Autodesk Inventor part; units mm, degrees
ref_plane "YZ Plane" through (0, 0, 0) normal (1, 0, 0) x (0, 1, 0)
ref_plane "XZ Plane" through (0, 0, 0) normal (0, 1, 0) x (-1, 0, 0)
ref_plane "XY Plane" through (0, 0, 0) normal (0, 0, 1) x (1, 0, 0)
sketch "Sketch1" plane through (0, 0, 0) normal (0, 0, 1) x (1, 0, 0)
  line L0 (-750, 62.1281) -> (750, 62.1281)
  line L1 (750, 62.1281) -> (750, 0)
  line L2 (750, 0) -> (-750, 0)
  line L3 (-750, 0) -> (-750, 62.1281)
  point P0 (0, 0)
  point P1 (0, 0)
  dimension "d0" = 1500
  dimension "d1" = 62.1281
extrude "Plate1" add sketch "Sketch1" along normal blind 3
sketch "Sketch2" plane through (750, 3, 0) normal (0, -1, 0) x (1, 0, 0)
  line L0 (-1500, 0) -> (0, 0)
  line L1 (0, 0) -> (0, 30)
  line L2 (0, 30) -> (-1500, 30)
  line L3 (-1500, 30) -> (-1500, 0)
edge flange "Flange1" height 30 angle 90 thickness 3 bend radius 3 thickness toward (0, -1, 0) relief tear relief width 3 relief depth 1.5 edges at (0, 0, 3) wall of the first edge with corners at (-750, 3, 0) (750, 3, 0) (750, 3, 30) (-750, 3, 30)
bend "Bend1"
corner "Corner1"
sketch "Sketch5" plane through (0, 0, 0) normal (0, 0, -1) x (-1, 0, 0)
  line L0 (750, 62.1281) -> (-750, 62.1281)
  line L1 (497, 62.1281) -> (497, 31)
  line L2 (497, 31) -> (500, 31)
  line L3 (500, 31) -> (500, 62.1281)
  line L4 (750, 0) -> (-750, 0)
  point P0 (0, 0)
  dimension "d18" = 3
  dimension "d19" = 250
  dimension "d20" = 31
extrude "Extrusion1" cut sketch "Sketch5" against normal through all
pattern_linear "Rectangular Pattern1" count 3 spacing 500 along (1, 0, 0) of "Extrusion1"
sketch "Sketch6" plane through (0, 0, 0) normal (0, 0, -1) x (-1, 0, 0)
  line L0 (-750, 62.1281) -> (-750, 6)
  circle A0 centre (-750, 62.1281) radius 15
  line L1 (-750, 62.1281) -> (-503, 62.1281)
  point P0 (0, 0)
  point P1 (-735, 62.1281)
  point P2 (-750, 47.1281)
  dimension "d24" = 30
extrude "Extrusion2" cut sketch "Sketch6" against normal through all contours L1 A0 L0 picked at (-740.1254, 61.0155)
mirror "Mirror1" about plane through (0, 0, 0) normal (1, 0, 0) of "Extrusion2"
equation "\"d1\" = Стрингер_2"
equation "\"d18\" = Thickness"
equation "\"d2\" = Thickness"
equation "\"d3\" = BendReliefWidth"
equation "\"d4\" = BendReliefDepth"
equation "\"d5\" = MinimumRemnant"
equation "\"d6\" = TransitionRadius"
equation "\"d9\" = BendRadius"
equation "\"d10\" = CornerReliefSize"
equation "\"d11\" = GapSize"
equation "\"d12\" = JacobiRadiusSize"
equation "\"BendRadius\" = Thickness"
equation "\"BendReliefWidth\" = Thickness"
equation "\"BendReliefDepth\" = 0.5 * Thickness"
equation "\"CornerReliefSize\" = 4 * Thickness"
equation "\"MinimumRemnant\" = 2 * Thickness"
equation "\"TransitionRadius\" = BendRadius"
equation "\"JacobiRadiusSize\" = BendRadius"
equation "\"GapSize\" = Thickness"
equation "\"qqqqqq\" = 67.35706"
properties part number "МОО 052 стрингер спина 2"
Design review of the part built by this model. Coordinates are the model's own, in mm. A direction names the side the tool comes from. Coordinates: 2 decimals unless noted, no trailing zeros. Order: outer loops, then holes, each group sorted by start corner. A loop starts at its lowest first (then second) coordinate and runs counter-clockwise, first axis right, second up. Notation, with made-up numbers: (-31, -17) - (23, -17) arc R23 cw to (23, -4) - close; hole circle Ø6 at (-22.75, -9). An arc over 180 degrees is marked (long way). Put each result on its own line as item: value.
1) Insertion check: P1, Ø0.9, axis at y = 50.5, z = 2, coming from the -X side; P2, Ø0.9, axis at x = 501.5, z = 1.5, coming from the +Y side; P3, Ø2, axis at x = -332.5, y = 20, coming from the +Z side; P4, Ø4, axis at y = 7.5, z = 6.5, coming from the +X side. Each pin has a flat end and moves straight along its axis. Give the tip position at first contact, or say it passes through.
Response values:
P1: stops at x = -741.11
P2: stops at y = 31
P3: stops at z = 3
P4: passes through
2) Tool access review of faces 1 (the face through (-10, 34, 0)), 2 (the face through (-10, 34, 3)): name each direction out of +Z, -Z, +X, -X, +Y, -Y from which nothing blocks a thin tool from reaching the whole face with its end or side.
Response values:
face 1: -Z, +X, -X, +Y, -Y
face 2: +Z, +X, -X, +Y
3) The part is to be moulded in two halves that separate along Y. For faces 3 (the face through (750, 16.5, 2.8)), 4 (the face through (10, 3, 18)), 5 (the face through (10, 0, 18)), say which applies: released by +Y, released by -Y, zero draft, split by the parting line, or undercut.
Response values:
face 3: zero draft
face 4: released by +Y
face 5: released by -Y
4) Take a section at A-A, the plane x = -347.5. Give the boundary of the cut face in (y, z).
Response values:
outline: (0, 6) arc R6 ccw to (6, 0) - (62.13, 0) - (62.13, 3) - (6, 3) arc R3 cw to (3, 6) - (3, 30) - (0, 30) - close
5) Take a section at B-B, the plane y = 16.5. Give the boundary of the cut face in (x, z), and give its area (3 significant figures).
Response values:
outline: (-750, 0) - (750, 0) - (750, 3) - (-750, 3) - close
area: 4,500 mm²
6) Wall thickness on L1, parallel to Z at x = 568.5, y = 37.5; L2, parallel to Z at x = 573.5, y = 4: over which ranges is each line inside the solid? List them lowest first. Write a range as from..to.
Response values:
L1: z = 0..3
L2: z = 0.34..3.76
